Autodesk Inventor part; units mm, degrees
ref_plane "YZ Plane" through (0, 0, 0) normal (1, 0, 0) x (0, 1, 0)
ref_plane "XZ Plane" through (0, 0, 0) normal (0, 1, 0) x (-1, 0, 0)
ref_plane "XY Plane" through (0, 0, 0) normal (0, 0, 1) x (1, 0, 0)
sketch "Sketch1" plane through (0, 0, 0) normal (0, 1, 0) x (-1, 0, 0)
  line L0 (4.825, 9.525) -> (-4.825, 9.525)
  line L1 (-4.825, 9.525) -> (-4.825, -9.525)
  line L2 (-4.825, -9.525) -> (4.825, -9.525)
  line L3 (4.825, -9.525) -> (4.825, 9.525)
  point P0 (0, 0)
  dimension "d0" = 9.65
  dimension "d1" = 4.825
  dimension "d2" = 19.05
  dimension "d3" = 9.525
extrude "Extrusion1" add sketch "Sketch1" along normal blind 4.83
sketch "Sketch2" plane through (0, 0, 0) normal (0, -1, 0) x (1, 0, 0)
  line L0 (5.715, 8.25) -> (3.935, 8.25)
  line L1 (3.935, 8.25) -> (3.935, 6.98)
  line L2 (3.935, 6.98) -> (5.715, 6.98)
  line L3 (5.715, 6.98) -> (5.715, 8.25)
  line L4 (-4.825, 9.525) -> (4.825, 9.525)
  line L5 (4.825, 9.525) -> (4.825, -9.525)
  line L6 (5.715, 7.87) -> (5.205, 7.87)
  line L7 (5.205, 7.36) -> (5.715, 7.36)
  line L8 (5.715, 7.36) -> (5.715, 7.87)
  line L9 (4.825, 8.25) -> (5.205, 7.87)
  line L10 (5.205, 7.36) -> (4.825, 6.98)
  point P0 (0, 0)
  dimension "d6" = 1.27
  dimension "d7" = 1.78
  dimension "d8" = 5.715
  dimension "d9" = 1.275
  dimension "d10" = 0.51
  dimension "d11" = 0.38
  dimension "d12" = 45
  dimension "d13" = 45
extrude "Extrusion2" add sketch "Sketch2" along normal blind 0.25 contours L5 L2 L1 L0 | L9 L6 L3 L7 L10 L5
pattern_linear "Rectangular Pattern1" count 4 spacing 5.08 along (0, 0, -1) of "Extrusion2"
mirror "Mirror1" about plane through (0, 0, 0) normal (1, 0, 0) of "Extrusion2", "Rectangular Pattern1"
properties part number "MC_YY101"
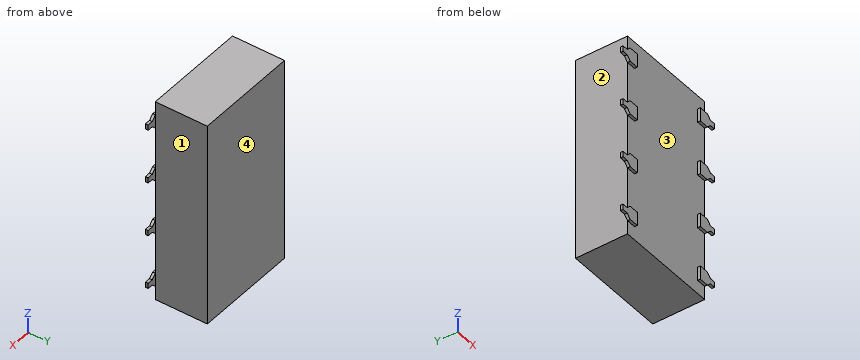
Design review of the part built by this model. Coordinates are the model's own, in mm. Face numbers are marked on the shaded views. Round coordinates to 2 decimals unless told otherwise and drop trailing zeros. Order: outer loops, then holes, each group sorted by start corner. A loop starts at its lowest first (then second) coordinate and runs counter-clockwise, first axis right, second up.
1) Draft analysis for pull direction X (two halves, no side actions). For the marked faces 1, 2, 3 and 4, state which applies: released by +X, released by -X, zero draft, split by the parting line, or undercut.
The answers:
face 1: released by +X
face 2: released by -X
face 3: undercut
face 4: zero draft
2) Consider section C-C (y = 3.1). State the section outline as (x, z) points (3 decimals).
The answers:
outline: (-4.825, -9.525) - (4.825, -9.525) - (4.825, 9.525) - (-4.825, 9.525) - close
3) Clearance check with flat-ended pins moving along their axes: pin 1 Ø2 at (y, z) = (1, 5.5) entering from +X (3 decimals); pin 2 Ø6 at (x, z) = (-3.5, -0.5) entering from -Y. State where each tip first meets the part, or that it passes through.
The answers:
pin 1: stops at x = 4.825
pin 2: stops at y = -0.25
4) For L1, parallel to X at y = 2.05, z = -1.75 (3 decimals); L2, parallel to Y at x = 0, z = -8.5, list the stretches that pass through material, from the lowest coordinate up.
The answers:
L1: x = -4.825 to 4.825
L2: y = 0 to 4.83
5) Consider section A-A (x = -4.25). State the section outline as (y, z) points (3 decimals).
The answers:
outline: (-0.25, -8.26) - (0, -8.26) - (0, -9.525) - (4.83, -9.525) - (4.83, 9.525) - (0, 9.525) - (0, 8.25) - (-0.25, 8.25) - (-0.25, 6.98) - (0, 6.98) - (0, 3.17) - (-0.25, 3.17) - (-0.25, 1.9) - (0, 1.9) - (0, -1.91) - (-0.25, -1.91) - (-0.25, -3.18) - (0, -3.18) - (0, -6.99) - (-0.25, -6.99) - close
6) Consider section B-B (z = 4.5). State the section outline as (x, y) points (3 decimals).
The answers:
outline: (-4.825, 0) - (4.825, 0) - (4.825, 4.83) - (-4.825, 4.83) - close
